Geometry check sheet. Reference: the model listing, model coordinates, mm. Face numbers are marked on the shaded views. A direction names the side the tool comes from. Give positions to 0.01 mm unless a question says otherwise; leave off trailing zeros. Write each loop counter-clockwise with the first axis right and the second up, starting at its lowest first coordinate (ties: lowest second). Pieces come first, ordered by that corner, then holes. Notation, with made-up numbers: M 51,41 L 92,41 A32 ccw 92,79 Z; hole C -33,52 d11. An arc over 180 degrees is marked long. One line per item, written item: value. Start each with the question number.
1. Cross-section at C-C on x = -8. Record the cut outline in (y, z).
2. Tool access check on the marked faces 5, 6, 7, 8 and 9. Record the directions out of +Z, -Z, +X, -X, +Y, -Y that give a thin tool (end or side, any length) a straight path to the whole face; none if there is none.
3. Gauge pin test, flat ends, axial feed: pin 1 (1.6 mm diameter, centred on y = 8.5, z = 2.5, fed in from -X); pin 2 (2 mm diameter, centred on y = -14, z = 3, fed in from +X); pin 3 (3 mm diameter, centred on x = 11, y = -1.5, fed in from -Z). Record the tip position at first contact, or that the pin passes through.
4. Cross-section at D-D on z = 1. Count the separate pieces of the cut face and the enclosed holes in it, then the cut area to 3 significant figures.
5. Release check for a two-part mould opening along Y. For the marked faces 1, 2, 3 and 4 record: pulls with the +Y half, pulls with the -Y half, needs draft (parallel to the pull), parting line crosses it, or undercut.
6. Cross-section at A-A on y = -4.25. Record the cut outline in (x, z), then the cut area to 3 significant figures.
7. Cross-section at B-B on x = -0.5. Record the cut outline in (y, z).
8. Scan lines: line 1 (X direction, y = -1.75, z = 1.5); line 2 (Y direction, x = 6.5, z = -1); line 3 (Y direction, x = 5.75, z = 7.75). Record each from-to range of solid material in increasing order.
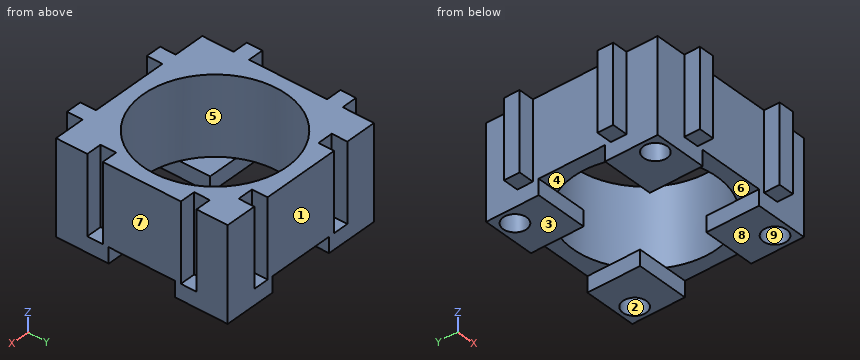
from build123d import *

# Parameters (mm, degrees)
SKETCH1_W           = 22
SKETCH1_H           = 22
BOSS_EXTRUDE1_DEPTH = 10
SKETCH3_W           = 2
SKETCH3_H           = 10
BOSS_EXTRUDE2_DEPTH = 2
SKETCH4_W           = 10
SKETCH4_H           = 2
BOSS_EXTRUDE3_DEPTH = 2
SKETCH5_W           = 10
SKETCH5_H           = 2
CUT_EXTRUDE1_DEPTH  = 2
SKETCH6_W           = 2
SKETCH6_H           = 10
CUT_EXTRUDE2_DEPTH  = 2
SKETCH7_R           = 9.2
CUT_EXTRUDE3_DEPTH  = 11
SKETCH8_W           = 6.75
SKETCH8_H           = 6.75
BOSS_EXTRUDE4_DEPTH = 2
SKETCH9_R           = 1.5
CUT_EXTRUDE6_DEPTH  = 6


with BuildPart() as part:
    # Sketch1 → Boss-Extrude1 (new body)
    with BuildSketch(Plane.XY):
        with Locations((1.600938967, -1.755868545)):
            Rectangle(SKETCH1_W, SKETCH1_H)
    extrude(amount=BOSS_EXTRUDE1_DEPTH)

    # Sketch3 → Boss-Extrude2 (add)
    with BuildSketch(Plane.XZ.offset(12.755868545)):
        with Locations((7.600938967, 5)):
            Rectangle(SKETCH3_W, SKETCH3_H)
        with Locations((-4.399061033, 5)):
            Rectangle(SKETCH3_W, SKETCH3_H)
    extrude(amount=BOSS_EXTRUDE2_DEPTH)

    # Sketch4 → Boss-Extrude3 (add)
    with BuildSketch(Plane.ZY.offset(9.399061033)):
        with Locations((5, 4.244131455)):
            Rectangle(SKETCH4_W, SKETCH4_H)
        with Locations((5, -7.755868545)):
            Rectangle(SKETCH4_W, SKETCH4_H)
    extrude(amount=BOSS_EXTRUDE3_DEPTH)

    # Sketch5 → Cut-Extrude1 (cut)
    with BuildSketch(Plane(origin=(12.600938967, 0, 0), x_dir=(0, 0, -1), z_dir=(1, 0, 0))):
        with Locations((-5, 4.244131455)):
            Rectangle(SKETCH5_W, SKETCH5_H)
        with Locations((-5, -7.755868545)):
            Rectangle(SKETCH5_W, SKETCH5_H)
    extrude(amount=-CUT_EXTRUDE1_DEPTH, mode=Mode.SUBTRACT)

    # Sketch6 → Cut-Extrude2 (cut)
    with BuildSketch(Plane(origin=(0, 9.244131455, 0), x_dir=(1, 0, 0), z_dir=(0, 1, 0))):
        with Locations((-4.399061033, -5)):
            Rectangle(SKETCH6_W, SKETCH6_H)
        with Locations((7.600938967, -5)):
            Rectangle(SKETCH6_W, SKETCH6_H)
    extrude(amount=-CUT_EXTRUDE2_DEPTH, mode=Mode.SUBTRACT)

    # Sketch7 → Cut-Extrude3 (cut, through all)
    with BuildSketch(Plane.XY.offset(10)):
        with Locations((1.600938967, -1.755868545)):
            Circle(SKETCH7_R)
    extrude(amount=-CUT_EXTRUDE3_DEPTH, mode=Mode.SUBTRACT)

    # Sketch8 → Boss-Extrude4 (add)
    with BuildSketch(Plane(origin=(0, 0, 0), x_dir=(-1, 0, 0), z_dir=(0, 0, -1))):
        with Locations((6.024061033, 5.869131455)):
            Rectangle(SKETCH8_W, SKETCH8_H)
        with Locations((-9.225938967, 5.869131455)):
            Rectangle(SKETCH8_W, SKETCH8_H)
        with Locations((-9.225938967, -9.380868545)):
            Rectangle(SKETCH8_W, SKETCH8_H)
        with Locations((6.024061033, -9.380868545)):
            Rectangle(SKETCH8_W, SKETCH8_H)
    extrude(amount=BOSS_EXTRUDE4_DEPTH)

    # Sketch9 → Cut-Extrude6 (cut)
    with BuildSketch(Plane(origin=(0, 0, -2), x_dir=(-1, 0, 0), z_dir=(0, 0, -1))):
        with Locations((7.399061033, -10.755868545)):
            Circle(SKETCH9_R)
        with Locations((-10.600938967, -10.755868545)):
            Circle(SKETCH9_R)
        with Locations((7.399061033, 7.244131455)):
            Circle(SKETCH9_R)
        with Locations((-10.600938967, 7.244131455)):
            Circle(SKETCH9_R)
    extrude(amount=-CUT_EXTRUDE6_DEPTH, mode=Mode.SUBTRACT)


solid = part.part
Report:
1. outline: M -12.76,-2 L -12.13,-2 L -12.13,4 L -9.38,4 L -9.38,-2 L -6.01,-2 L -6.01,0 L 2.49,0 L 2.49,-2 L 5.87,-2 L 5.87,4 L 8.62,4 L 8.62,-2 L 9.24,-2 L 9.24,10 L -12.76,10 Z
2. face 5: +Z
2. face 6: -Z, +Y, -Y
2. face 7: +Z, -Z, +X, +Y, -Y
2. face 8: -Z, +X, -X, +Y, -Y
2. face 9: -Z
3. pin 1: stops at x = -9.4
3. pin 2: stops at x = 8.6
3. pin 3: stops at z = 0
4. separate pieces: 1
4. enclosed holes: 5
4. area: 190 mm^2
5. face 1: pulls with the +Y half
5. face 2: undercut
5. face 3: needs draft
5. face 4: undercut
6. outline: M -9.4,0 L -7.25,0 L -7.25,10 L -9.4,10 Z; M 10.46,0 L 12.6,0 L 12.6,10 L 10.46,10 Z
6. area: 42.9 mm^2
7. outline: M -12.76,0 L -10.71,0 L -10.71,10 L -12.76,10 Z; M 7.2,0 L 9.24,0 L 9.24,10 L 7.2,10 Z
8. line 1: x = -9.4 to -7.6, 10.8 to 12.6
8. line 2: y = -12.76 to -6.01, 2.49 to 9.24
8. line 3: y = -12.76 to -9.97, 6.46 to 9.24
